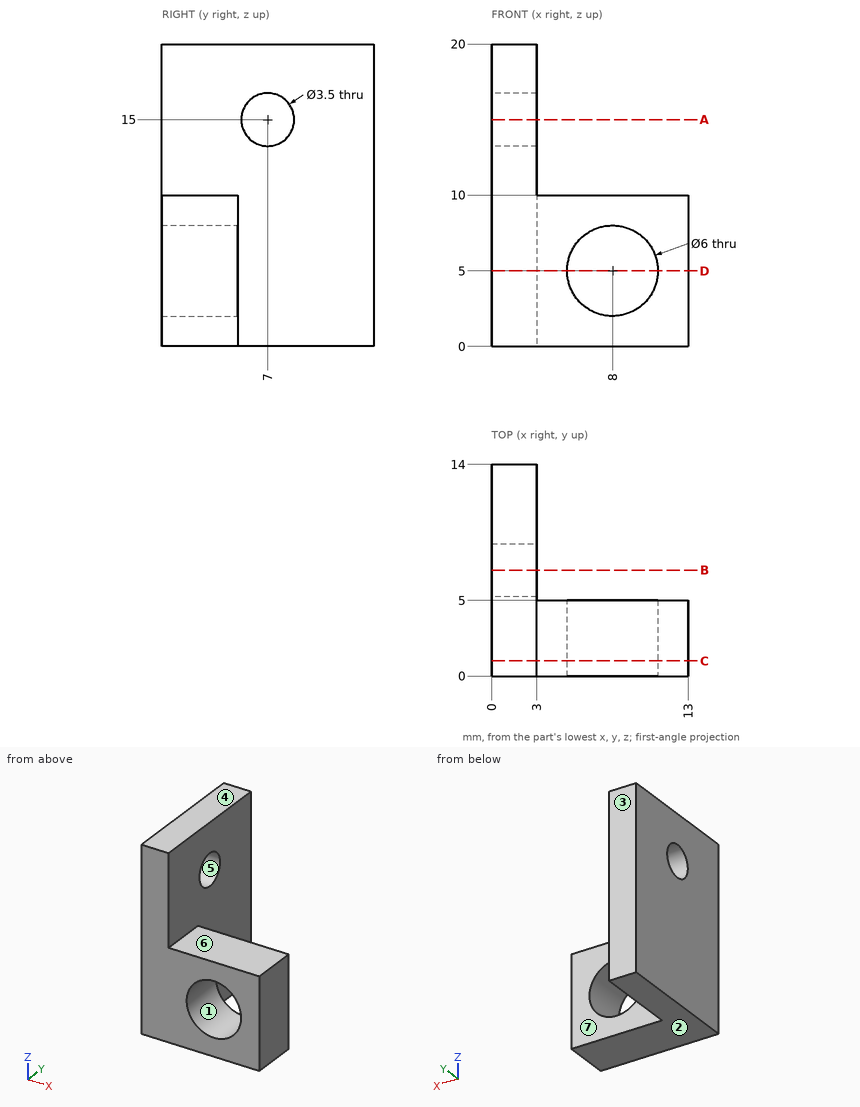
Check sheet for the drawn part. Datum: minimum x, y, z corner. Units: mm. A direction names the side the tool comes from. Give positions to 0.01 mm unless a question says otherwise; leave off trailing zeros. Order: outer loops, then holes, each group sorted by start corner. A loop starts at its lowest first (then second) coordinate and runs counter-clockwise, first axis right, second up. Notation, with made-up numbers: (-2.5, 50) -> (29.5, 50) arc R21 ccw to (29.5, 87) -> close; hole circle Ø11 at (-13.75, 79.25). An arc over 180 degrees is marked (long way). One line per item, written item: value.
(1) Sectioned sample at D-D on z = 5. Record the cut outline in (x, y), then the cut area to 3 significant figures.
Final values:
outline: (0, 0) -> (5, 0) -> (5, 5) -> (3, 5) -> (3, 14) -> (0, 14) -> close; (11, 0) -> (13, 0) -> (13, 5) -> (11, 5) -> close
area: 62.0 mm^2
(2) Sectioned sample at C-C on y = 1. Record the cut outline in (x, z), then the cut area to 3 significant figures.
Final values:
outline: (0, 0) -> (13, 0) -> (13, 10) -> (3, 10) -> (3, 20) -> (0, 20) -> close; hole circle Ø6 at (8, 5)
area: 132 mm^2
(3) Scan lines: line 1 along X through (y, z) = (3.65, 5); line 2 along Z through (x, y) = (2.1, 7); line 3 along Z through (x, y) = (8, 2.95). Record each from-to range of solid material in increasing order. Write a range as [from, to].
Final values:
line 1: [0, 5], [11, 13]
line 2: [0, 13.25], [16.75, 20]
line 3: [0, 2], [8, 10]
(4) Tool access check on the marked faces 5, 6 and 7. Record the directions out of +Z, -Z, +X, -X, +Y, -Y that give a thin tool (end or side, any length) a straight path to the whole face; none if there is none.
Final values:
face 5: +X, -X
face 6: +Z, +X, +Y, -Y
face 7: +Z, -Z, +X, +Y
(5) Draft check along Z on the marked faces 1, 2, 3 and 4. Enter one of: pulls with the +Z half, pulls with the -Z half, needs draft (parallel to the pull), parting line crosses it, or undercut.
Final values:
face 1: undercut
face 2: pulls with the -Z half
face 3: needs draft
face 4: pulls with the +Z half
(6) Sectioned sample at B-B on y = 7. Record the cut outline in (x, z), then the cut area to 3 significant figures.
Final values:
outline: (0, 0) -> (3, 0) -> (3, 13.25) -> (0, 13.25) -> close; (0, 16.75) -> (3, 16.75) -> (3, 20) -> (0, 20) -> close
area: 49.5 mm^2
(7) Sectioned sample at A-A on z = 15. Record the cut outline in (x, y).
Final values:
outline: (0, 0) -> (3, 0) -> (3, 5.25) -> (0, 5.25) -> close; (0, 8.75) -> (3, 8.75) -> (3, 14) -> (0, 14) -> close
(8) Gauge pin test, flat ends, axial feed: pin 1 (5.5 mm diameter, centred on y = 7, z = 15, fed in from +X); pin 2 (3 mm diameter, centred on x = 10, z = 4, fed in from +Y); pin 3 (5.5 mm diameter, centred on x = 7, y = 2.5, fed in from +Z). Record the tip position at first contact, or that the pin passes through.
Final values:
pin 1: x = 3
pin 2: y = 5
pin 3: z = 10
